Can you work these out from the model? Positions are in its coordinate system, mm. Face numbers are marked on the shaded views. A direction names the side the tool comes from. Coordinates: 2 decimals unless noted, no trailing zeros. Loops run counter-clockwise (first coordinate to the right, second up) from the corner with the lowest first, then second, coordinate; pieces in that order, holes last. Notation, with made-up numbers: (11.5, 88) -> (49.5, 88) arc R16 ccw to (49.5, 95) -> close; hole circle Ø2 at (-34, -18). An arc over 180 degrees is marked (long way). Put each result on its own line as item: value. Start each with the question number.
Item 1: If we section it at D-D on y = -11.6: Please give me the cut outline in (x, z).
Item 2: If we section it at A-A on z = 6: Please give me the cut outline in (x, y).
Item 3: Will these pins go through, and if not, where does the flat tip stop? P1, Ø3, axis at x = 4.5, y = 3.5, coming from the -Z side; P2, Ø4, axis at x = 11.6, y = 11.6, coming from the +Z side; P3, Ø1, axis at x = 8.5, z = 12, coming from the +Y side.
Item 4: For the marked faces 1, 2 and 3, which set-ups out of +Z, -Z, +X, -X, +Y, -Y let a thin tool reach every point of the face, with its end or its side?
Item 5: If we section it at B-B on x = 0: Please give me the cut outline in (y, z), plus the area to 3 significant figures.
Item 6: Please list where these lines run through material, in increasing order: L1, parallel to Y at x = -11.6, z = 3; L2, parallel to X at y = 11, z = 6.75; L3, parallel to Y at x = -10.5, z = 8.25. Write a range as from..to.
```python
from build123d import *

# Parameters (mm, degrees)
SKETCH_1_W               = 28
SKETCH_1_H               = 28
EXTRUDE_1_DEPTH          = 10
SKETCH_2_R               = 6.5
CUT_EXTRUDE_1_DEPTH      = 11
SKETCH_3_R               = 7.55
CUT_EXTRUDE_2_DEPTH      = 6
SKETCH_6_R               = 11.05
CUT_EXTRUDE_3_DEPTH      = 2
FILLET_1_R               = 2
SKETCH_7_W               = 0.995329216
SKETCH_7_H               = 2
EXTRUDE_2_DEPTH          = 3
PATTERN_CIRCULAR_1_COUNT = 4
SKETCH_8_R               = 12
CUT_EXTRUDE_4_DEPTH      = 3
SKETCH_9_R               = 1.3
CUT_EXTRUDE_5_DEPTH      = 14


with BuildPart() as part:
    # 草图1 → 凸台-拉伸1 (new body)
    with BuildSketch(Plane.XY):
        Rectangle(SKETCH_1_W, SKETCH_1_H)
    extrude(amount=EXTRUDE_1_DEPTH)

    # 草图2 → 切除-拉伸1 (cut, through all)
    with BuildSketch(Plane.XY.offset(10)):
        Circle(SKETCH_2_R)
    extrude(amount=-CUT_EXTRUDE_1_DEPTH, mode=Mode.SUBTRACT)

    # 草图3 → 切除-拉伸2 (cut)
    with BuildSketch(Plane.XY.offset(10)):
        Circle(SKETCH_3_R)
    extrude(amount=-CUT_EXTRUDE_2_DEPTH, mode=Mode.SUBTRACT)

    # 草图6 → 切除-拉伸3 (cut)
    with BuildSketch(Plane(origin=(0, 0, 0), x_dir=(-1, 0, 0), z_dir=(0, 0, -1))):
        Circle(SKETCH_6_R)
    extrude(amount=-CUT_EXTRUDE_3_DEPTH, mode=Mode.SUBTRACT)

    # 圆角1
    fillet_1_edges = [part.edges().sort_by_distance(p)[0] for p in [
        (14, -14, 5),
        (-14, -14, 5),
        (-14, 14, 5),
        (14, 14, 5),
    ]]
    fillet(fillet_1_edges, radius=FILLET_1_R)

    # 草图7 → 凸台-拉伸2 (add)
    with BuildSketch(Plane.XY.offset(10)):
        with Locations((-13.502335392, -8)):
            Rectangle(SKETCH_7_W, SKETCH_7_H)
    extrude_2 = extrude(amount=EXTRUDE_2_DEPTH)

    # 阵列(圆周)1: 凸台-拉伸2 ×4 about axis
    pattern_circular_1_axis = Axis((0, 0, 0), (0, 0, 1))
    for i in range(1, PATTERN_CIRCULAR_1_COUNT):
        add(extrude_2.rotate(pattern_circular_1_axis, i * 360 / PATTERN_CIRCULAR_1_COUNT))

    # 草图8 → 切除-拉伸4 (cut)
    with BuildSketch(Plane.XY.offset(10)):
        Circle(SKETCH_8_R)
    extrude(amount=-CUT_EXTRUDE_4_DEPTH, mode=Mode.SUBTRACT)

    # 草图9 → 切除-拉伸5 (cut, through all)
    with BuildSketch(Plane(origin=(0, 0, 0), x_dir=(-1, 0, 0), z_dir=(0, 0, -1))):
        with Locations((-11.6, 11.6)):
            Circle(SKETCH_9_R)
        with Locations((11.6, 11.6)):
            Circle(SKETCH_9_R)
        with Locations((11.6, -11.6)):
            Circle(SKETCH_9_R)
        with Locations((-11.6, -11.6)):
            Circle(SKETCH_9_R)
    extrude(amount=-CUT_EXTRUDE_5_DEPTH, mode=Mode.SUBTRACT)


solid = part.part
```
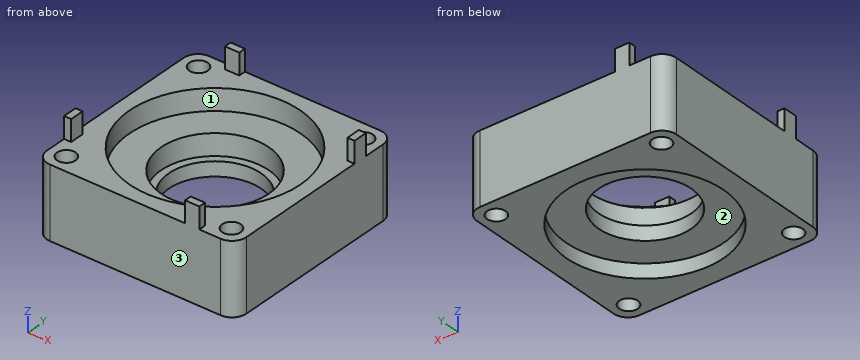
Solutions:
1. outline: (-14, 0) -> (-12.9, 0) -> (-12.9, 10) -> (-14, 10) -> close; (-10.3, 0) -> (10.3, 0) -> (10.3, 10) -> (3.07, 10) -> (3.07, 7) -> (-3.07, 7) -> (-3.07, 10) -> (-10.3, 10) -> close; (12.9, 0) -> (14, 0) -> (14, 10) -> (12.9, 10) -> close
2. outline: (-14, -12) arc R2 ccw to (-12, -14) -> (12, -14) arc R2 ccw to (14, -12) -> (14, 12) arc R2 ccw to (12, 14) -> (-12, 14) arc R2 ccw to (-14, 12) -> close; hole circle Ø2.6 at (-11.6, -11.6); hole circle Ø2.6 at (-11.6, 11.6); hole circle Ø15.1 at (0, 0); hole circle Ø2.6 at (11.6, -11.6); hole circle Ø2.6 at (11.6, 11.6)
3. P1: z = 2
3. P2: z = 10
3. P3: y = -13
4. face 1: +Z
4. face 2: -Z
4. face 3: +Z, -Z, +X, -X, -Y
5. outline: (-14, 0) -> (-11.05, 0) -> (-11.05, 2) -> (-6.5, 2) -> (-6.5, 4) -> (-7.55, 4) -> (-7.55, 7) -> (-12, 7) -> (-12, 10) -> (-14, 10) -> close; (6.5, 2) -> (11.05, 2) -> (11.05, 0) -> (14, 0) -> (14, 10) -> (12, 10) -> (12, 7) -> (7.55, 7) -> (7.55, 4) -> (6.5, 4) -> close
5. area: 92.5 mm^2
6. L1: -14..-12.9, -10.3..10.3, 12.9..14
6. L2: -14..-12.75, -10.45..10.45, 12.75..14
6. L3: -14..-12.29, -10.91..-5.81, 5.81..10.91, 12.29..14
